Geometry check sheet. Reference: the model listing, model coordinates, mm. A direction names the side the tool comes from. Round coordinates to 2 decimals unless told otherwise and drop trailing zeros. Loops run counter-clockwise (first coordinate to the right, second up) from the corner with the lowest first, then second, coordinate; pieces in that order, holes last.
Autodesk Fusion 360 part; units mm, degrees
sketch "Sketch1" plane through (0, 0, 0) normal (0, 1, 0) x (1, 0, 0)
  line L0 (0, 0) -> (60, 0)
  line L1 (0, 0) -> (-60, 0)
  line L2 (-60, 0) -> (-60, 15)
  line L3 (-60, 15) -> (-40, 15)
  line L4 (30, 10) -> (-30, 10)
  line L5 (40, 15) -> (60, 15)
  line L6 (60, 15) -> (60, 0)
  line L7 (-40, 15) -> (-30, 15)
  line L8 (-30, 15) -> (-30, 10)
  line L9 (30, 10) -> (30, 15)
  line L10 (40, 15) -> (30, 15)
  line L11 (60, 0) -> (30, 0)
  line L12 (30, 0) -> (35, 0)
  line L13 (35, 0) -> (25, 0)
  line L14 (25, 0) -> (25, -25.359)
  line L15 (35, -25.359) -> (35, 0)
  arc A0 (25, -25.359) -> (35, -25.359) centre (30, -60) ccw
  circle A1 centre (30, -60) radius 25
  line L16 (25, 0) -> (-30, 0)
  line L17 (-60, 0) -> (-25, 0)
  line L18 (-25, 0) -> (-3.4631, -70.2578)
extrude "Extrude1" add sketch "Sketch1" along normal blind 40 contours L0 L1 L2 L3 L4 L5 L6 L7 L8 L9 L10 L11 L12 L13 L16 L17
extrude "Extrude3" add sketch "Sketch1" along normal blind 30 contours L0 L11 L12 L13 L14 L15 A0
extrude "Extrude2" add sketch "Sketch1" along normal blind 5 contours L0 L1 L14 A0 L16 L18
sketch "Sketch2" plane through (0, 0, 0) normal (0, 0, 1) x (-1, 0, 0)
  line L0 (25, -5) -> (-25, -5)
  line L1 (-25, -5) -> (-25, -30)
  line L2 (-25, -30) -> (-35, -30)
  line L3 (-35, -30) -> (-35, 0)
  line L4 (-35, 0) -> (-60, 0)
  line L5 (-60, 0) -> (-60, -40)
  line L6 (-60, -40) -> (60, -40)
  line L7 (60, -40) -> (60, 0)
  line L8 (60, 0) -> (25, 0)
  line L9 (25, 0) -> (25, -5)
  line L10 (-60, -40) -> (-45, -40)
  line L11 (-45, -40) -> (-45, -25)
  circle A0 centre (-45, -25) radius 5
  line L12 (60, -40) -> (60, -25)
  line L13 (60, -25) -> (45, -25)
  circle A1 centre (45, -25) radius 5
  dimension "d7" = 10
  dimension "d8" = 10
extrude "Extrude4" cut sketch "Sketch2" against normal blind 15 contours A0 | A1
mirror "Mirror1" about plane through (0, 0, 0) normal (0, -1, 0) of bodies 1 merged
1) Sectioned sample at B-B, the plane x = -45. Record the cut outline in (y, z).
Report:
outline: (-40, -15) - (-30, -15) - (-30, 0) - (-40, 0) - close; (-20, -15) - (20, -15) - (20, 0) - (-20, 0) - close; (30, -15) - (40, -15) - (40, 0) - (30, 0) - close
2) Gauge pin test, flat ends, axial feed: pin 1 (5 mm diameter, centred on y = -12.5, z = 64, fed in from -X); pin 2 (8 mm diameter, centred on x = -45, y = -25, fed in from +Z); pin 3 (11.5 mm diameter, centred on x = -45, y = 25, fed in from +Z); pin 4 (13 mm diameter, centred on x = 45, y = -25, fed in from +Z). Record the tip position at first contact, or that the pin passes through.
Report:
pin 1: stops at x = -4.97
pin 2: passes through
pin 3: stops at z = 0
pin 4: stops at z = 93.95
3) Mould release check, pull along Z, two halves, no side actions. Record for faces 1 (the face through (-30, -1, -13)), 2 (the face through (-45, -1, -15)), 3 (the face through (0, 5, 19)): +Z half, -Z half, draft (parallel to the pull), parting line (faces both ways), or undercut.
Report:
face 1: draft
face 2: -Z half
face 3: undercut
4) Sectioned sample at D-D, the plane y = 15. Record the cut outline in (x, z), then the cut area to 3 significant figures.
Report:
outline: (-60, -15) - (-30, -15) - (-30, -10) - (30, -10) - (30, -15) - (60, -15) - (60, 0) - (35, 0) - (35, 25.36) arc R35 ccw (long way) to (25, 25.36) - (25, 0) - (-60, 0) - close; hole circle Ø50 at (30, 60)
area: 3,640 mm2
5) Sectioned sample at C-C, the plane x = 45. Record the cut outline in (y, z).
Report:
outline: (-40, -15) - (-30, -15) - (-30, 0) - (-40, 0) - close; (-30, 28.38) - (30, 28.38) - (30, 40) - (-30, 40) - close; (-30, 80) - (30, 80) - (30, 91.62) - (-30, 91.62) - close; (-20, -15) - (20, -15) - (20, 0) - (-20, 0) - close; (30, -15) - (40, -15) - (40, 0) - (30, 0) - close
6) Sectioned sample at A-A, the plane y = -25. Record the cut outline in (x, z).
Report:
outline: (-60, -15) - (-50, -15) - (-50, 0) - (-60, 0) - close; (-40, -15) - (-30, -15) - (-30, -10) - (30, -10) - (30, -15) - (40, -15) - (40, 0) - (35, 0) - (35, 25.36) arc R35 ccw (long way) to (25, 25.36) - (25, 0) - (-40, 0) - close; (50, -15) - (60, -15) - (60, 0) - (50, 0) - close; hole circle Ø50 at (30, 60)
7) Scan lines: line 1 along Y through (x, z) = (45, -4.5); line 2 along X through (y, z) = (25, -4.5); line 3 along Z through (x, y) = (15, 17). Record each from-to range of solid material in increasing order.
Report:
line 1: y = -40 to -30, -20 to 20, 30 to 40
line 2: x = -60 to -50, -40 to 40, 50 to 60
line 3: z = -10 to 0, 28.38 to 40, 80 to 91.62
8) Access from +Z, -Z, +X, -X, +Y, -Y to the whole of each face (thin tool, end or side, straight path). Record for faces 4 (the face through (35, 0, 13)), 5 (the face through (40.2, 30, 36.7)), 6 (the face through (1, -9, 0)), 7 (the face through (19.8, -30, 36.7)), 8 (the face through (25, -17, 13)).
Report:
face 4: +X, +Y, -Y
face 5: +Z, +X, -X, +Y
face 6: none
face 7: +Z, +X, -X, -Y
face 8: -X, -Y
